Design review of the part built by this model. Coordinates are the model's own, in mm. Give positions to 0.01 mm unless a question says otherwise; leave off trailing zeros. Write each loop counter-clockwise with the first axis right and the second up, starting at its lowest first coordinate (ties: lowest second). Pieces come first, ordered by that corner, then holes. Notation, with made-up numbers: M 73.5,70.25 L 77.5,70.25 A18 ccw 77.5,95.25 Z; hole C 77.25,33.5 d5. An arc over 180 degrees is marked long. Write each question's results on one line, items separated by ' | '. Start each with the question number.
from build123d import *

# Parameters (mm, degrees)
F1_DEPTH = 12.7
F2_SIZE2 = 38.1
F2_SIZE  = 38.1
F4_D     = 6.35
F6_D     = 3.96875
F7_D     = 8.7376


with BuildPart() as f1:
    # F0 (on Front) → F1 (new body)
    with BuildSketch(Plane.XZ):
        with BuildLine():
            Line((711.2, 78.1812), (711.2, 0))
            Line((711.2, 0), (1473.2, 0))
            Line((1473.2, 0), (1473.2, 562.7624))
            Line((1473.2, 562.7624), (711.2, 562.7624))
            Line((711.2, 562.7624), (711.2, 484.5812))
            ThreePointArc((711.2, 484.5812), (688.881537, 430.699663), (635, 408.3812))
            Line((635, 408.3812), (0, 408.3812))
            Line((0, 408.3812), (0, 154.3812))
            Line((0, 154.3812), (635, 154.3812))
            ThreePointArc((635, 154.3812), (688.881537, 132.062737), (711.2, 78.1812))
        make_face()
    extrude(amount=F1_DEPTH)

    # F2
    f2_edges = [f1.edges().sort_by_distance(p)[0] for p in [
        (711.2, -6.35, 562.7624),
        (711.2, -6.35, 0),
        (1473.2, -6.35, 0),
        (1473.2, -6.35, 562.7624),
        (0, -6.35, 154.3812),
        (0, -6.35, 408.3812),
    ]]
    chamfer(f2_edges, length=F2_SIZE, length2=F2_SIZE2)

    # F4 (through all)
    with Locations(Plane.XZ.offset(12.7)):
        with Locations((1092.2, 215.9), (1092.2, 346.8624), (1282.7, 346.8624), (1282.7, 215.9)):
            Hole(F4_D / 2)

    # F6 (through all)
    with Locations(Plane.XZ.offset(12.7)):
        with Locations((749.293897, 545.3126), (749.293897, 502.4374), (774.693897, 502.4374), (774.693897, 545.3126), (749.293897, 60.325), (774.693897, 17.4498), (749.293897, 17.4498), (774.693897, 60.325), (1409.706103, 502.4374), (1435.106103, 502.4374), (1435.106103, 545.3126), (1409.706103, 545.3126), (1409.706103, 17.4498), (1435.106103, 17.4498), (1435.106103, 60.325), (1409.706103, 60.325)):
            Hole(F6_D / 2)

    # F7 (through all)
    with Locations(Plane.XZ.offset(12.7)):
        with Locations((12.7, 370.1542), (50.8, 370.1542), (12.7, 192.6082), (50.8, 192.6082), (711.2, 370.1542), (749.3, 370.1542), (711.2, 192.6082), (749.3, 192.6082)):
            Hole(F7_D / 2)


solid = f1.part
Q1. For pin 1 Ø4.5 at (x, z) = (1435.11, 545.31) entering from +Y; pin 2 Ø6.5 at (x, y) = (401.5, -6) entering from +Z; pin 3 Ø2 at (y, z) = (-5, 406) entering from -X; pin 4 Ø1.5 at (x, y) = (391.5, -7.5) entering from -Z, all flat-tipped, find the tip position at first contact; note any pin that passes through.
Q2. We need section A-A on x = 499.5. Write out the cut boundary in (y, z).
Q3. We need section C-C on x = 690.5. Write out the cut boundary in (y, z).
Q4. Wall thickness on line 1 along Z through (x, y) = (1282.7, -2.25) (3 decimals); line 2 along Z through (x, y) = (12.7, -2.25); line 3 along Z through (x, y) = (621, -2.5): over which ranges is each line inside the solid? List them lowest first. Write a range as from..to.
Q5. We need section B-B on y = -6.75. Count the separate pieces of the cut face and the enclosed holes in it, and give its area (3 significant figures).
Answer sheet:
1) pin 1: y = 0 | pin 2: z = 408.38 | pin 3: x = 34.72 | pin 4: z = 154.38
2) outline: M -12.7,154.38 L 0,154.38 L 0,408.38 L -12.7,408.38 Z
3) outline: M -12.7,130.39 L 0,130.39 L 0,432.37 L -12.7,432.37 Z
4) line 1: 0..212.725, 219.075..343.687, 350.037..562.762 | line 2: 179.78..188.24, 196.98..365.79, 374.52..382.98 | line 3: 154.38..408.38
5) separate pieces: 1 | enclosed holes: 28 | area: 607,000 mm^2
